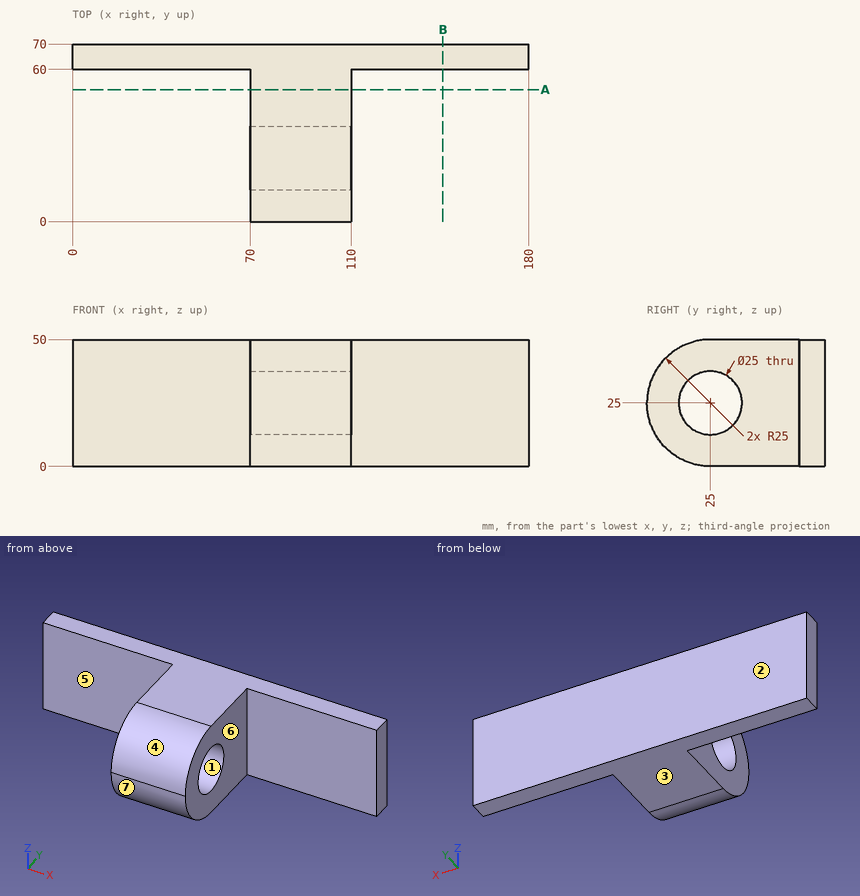
Could you check a few things on this drawing? It's one solid part, dimensions in mm from its lowest x, y, z. A direction names the side the tool comes from. Give positions to 0.01 mm unless a question says otherwise; leave off trailing zeros. Order: outer loops, then holes, each group sorted by start corner. A loop starts at its lowest first (then second) coordinate and runs counter-clockwise, first axis right, second up. Notation, with made-up numbers: (-32.75, 85) -> (-24.75, 85) arc R20 cw to (-24.75, 95) -> close; hole circle Ø11 at (9, 88.5). An arc over 180 degrees is marked (long way). Answer in a Markdown table with one row per item. Add a question column.
Item 1: Imagine slicing it at B-B (x = 146). List the corners of the cut face in (y, z) for me.
Item 2: Please list where these lines run through material, in increasing order: probe 1 along Y at (x, z) = (83.5, 25); probe 2 along Y at (x, z) = (55, 25.5); probe 3 along X at (y, z) = (58.5, 29).
Item 3: For the marked faces 5, 6 and 7, which set-ups out of +Z, -Z, +X, -X, +Y, -Y let a thin tool reach every point of the face, with its end or its side?
Item 4: We'd pull the mould along Z, two halves only. Please class the marked faces 1, 2, 3 and 4: pulls with the +Z half, pulls with the -Z half, needs draft (parallel to the pull), parting line crosses it, or undercut.
Item 5: Imagine slicing it at A-A (y = 52). List the corners of the cut face in (x, z) for me.
Item 6: I'm going to push flat-ended pins straight in: P1, Ø5, axis at x = 145.5, z = 37.5, coming from the -Y side; P2, Ø5, axis at y = 42, z = 7.5, coming from the +X side; P3, Ø1.5, axis at y = 40.5, z = 27.5, coming from the -X side. Where does each tip first touch, or does it pass through?
Result:
| question | item | result |
|---|---|---|
| 1 | outline | (60, 0) -> (70, 0) -> (70, 50) -> (60, 50) -> close |
| 2 | probe 1 | 0 to 12.5, 37.5 to 70 |
| 2 | probe 2 | 60 to 70 |
| 2 | probe 3 | 70 to 110 |
| 3 | face 5 | +Z, -Z, -X, -Y |
| 3 | face 6 | +Z, -Z, +X, -Y |
| 3 | face 7 | -Z, +X, -X, -Y |
| 4 | face 1 | undercut |
| 4 | face 2 | needs draft |
| 4 | face 3 | pulls with the -Z half |
| 4 | face 4 | pulls with the +Z half |
| 5 | outline | (70, 0) -> (110, 0) -> (110, 50) -> (70, 50) -> close |
| 6 | P1 | y = 60 |
| 6 | P2 | x = 110 |
| 6 | P3 | x = 70 |
